Verification items for the finished model (mm, model axes). Face numbers are marked on the shaded views. Give positions to 0.01 mm unless a question says otherwise; leave off trailing zeros. Order: outer loops, then holes, each group sorted by start corner. A loop starts at its lowest first (then second) coordinate and runs counter-clockwise, first axis right, second up. Notation, with made-up numbers: (-24, 87) - (-12, 87) arc R9 ccw to (-12, 97) - close; hole circle Ø6 at (89.5, 89.5). An arc over 180 degrees is marked (long way). Answer as a JSON object with one key per item and string values.
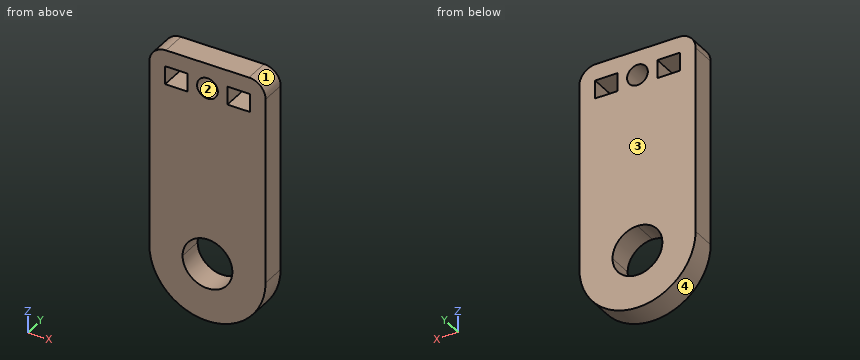
```python
from build123d import *

# Parameters (mm, degrees)
EXTRUDE_2_DEPTH = 3
SKETCH_1_4_W    = 2.7
SKETCH_1_4_H    = 2.2
SKETCH_1_4_R    = 1.25
EXTRUDE_3_DEPTH = 3
FILLET_2_R      = 2


with BuildPart() as part:
    # Sketch 1 → Extrude 2 (new body)
    with BuildSketch(Plane(origin=(0, 0, 0), x_dir=(1, 0, 0), z_dir=(0, 1, 0))):
        with BuildLine():
            ThreePointArc((-3, 12.25), (0, 15.25), (3, 12.25))
            Line((3, 12.25), (7, 12.25))
            ThreePointArc((7, 12.25), (0, 19.25), (-7, 12.25))
            Line((-7, 12.25), (-3, 12.25))
        make_face()
        with BuildLine():
            ThreePointArc((3, 12.25), (2.121320344, 10.128679656), (0, 9.25))
            Line((0, 9.25), (0, 5.25))
            ThreePointArc((0, 5.25), (4.949747468, 7.300252532), (7, 12.25))
            Line((7, 12.25), (3, 12.25))
        make_face()
        with BuildLine():
            Line((0, 5.25), (0, 9.25))
            ThreePointArc((0, 9.25), (-2.121320344, 10.128679656), (-3, 12.25))
            Line((-3, 12.25), (-7, 12.25))
            ThreePointArc((-7, 12.25), (-4.949747468, 7.300252532), (0, 5.25))
        make_face()
    extrude(amount=EXTRUDE_2_DEPTH)

    # Sketch 1_4 → Extrude 3 (add)
    with BuildSketch(Plane(origin=(0, 0, 0), x_dir=(1, 0, 0), z_dir=(0, 1, 0))):
        with BuildLine():
            ThreePointArc((7, 12.25), (4.949747468, 7.300252532), (0, 5.25))
            ThreePointArc((0, 5.25), (-4.949747468, 7.300252532), (-7, 12.25))
            Line((-7, 12.25), (-7, -12.25))
            Line((-7, -12.25), (7, -12.25))
            Line((7, -12.25), (7, 12.25))
        make_face()
        with Locations((-3.75, -9.170716156)):
            Rectangle(SKETCH_1_4_W, SKETCH_1_4_H, mode=Mode.SUBTRACT)
        with Locations((0, -9.25)):
            Circle(SKETCH_1_4_R, mode=Mode.SUBTRACT)
        with Locations((3.75, -9.170716156)):
            Rectangle(SKETCH_1_4_W, SKETCH_1_4_H, mode=Mode.SUBTRACT)
    extrude(amount=EXTRUDE_3_DEPTH)

    # Fillet 2
    fillet_2_edges = [part.edges().sort_by_distance(p)[0] for p in [
        (-7, 1.5, 12.25),
        (7, 1.5, 12.25),
    ]]
    fillet(fillet_2_edges, radius=FILLET_2_R)


solid = part.part
```
(1) Section check D-D (z = -10). Record the cut outline in (x, y), then the cut area to 3 significant figures.
Computed values:
{"outline": "(-7, 0) - (-1.98, 0) - (-1.98, 3) - (-7, 3) - close; (1.98, 0) - (7, 0) - (7, 3) - (1.98, 3) - close", "area": "30.1 mm²"}
(2) Release check for a two-part mould opening along X. For the marked faces 1, 2, 3 and 4 record: pulls with the +X half, pulls with the -X half, needs draft (parallel to the pull), parting line crosses it, or undercut.
Computed values:
{"face 1": "pulls with the +X half", "face 2": "undercut", "face 3": "needs draft", "face 4": "parting line crosses it"}
(3) Section check B-B (y = 2). Record the cut outline in (x, z), then the cut area to 3 significant figures.
Computed values:
{"outline": "(-7, -12.25) arc R7 ccw to (7, -12.25) - (7, 10.25) arc R2 ccw to (5, 12.25) - (-5, 12.25) arc R2 ccw to (-7, 10.25) - close; hole (-5.1, 8.07) - (-2.4, 8.07) - (-2.4, 10.27) - (-5.1, 10.27) - close; hole circle Ø6 at (0, -12.25); hole circle Ø2.5 at (0, 9.25); hole (2.4, 8.07) - (5.1, 8.07) - (5.1, 10.27) - (2.4, 10.27) - close", "area": "373 mm²"}
(4) Section check C-C (x = 0.5). Record the cut outline in (y, z), then the cut area to 3 significant figures.
Computed values:
{"outline": "(0, -19.23) - (3, -19.23) - (3, -15.21) - (0, -15.21) - close; (0, -9.29) - (3, -9.29) - (3, 8.1) - (0, 8.1) - close; (0, 10.4) - (3, 10.4) - (3, 12.25) - (0, 12.25) - close", "area": "69.8 mm²"}
(5) Material ranges on line 1 along Z through (x, y) = (0, 1.15); line 2 along X through (y, z) = (1.85, 9.25); line 3 along Z through (x, y) = (-1, 2.6), recorded low to high. Write a range as [from, to].
Computed values:
{"line 1": "z = [-19.25, -15.25], [-9.25, 8], [10.5, 12.25]", "line 2": "x = [-7, -5.1], [-2.4, -1.25], [1.25, 2.4], [5.1, 7]", "line 3": "z = [-19.18, -15.08], [-9.42, 8.5], [10, 12.25]"}
(6) Section check A-A (z = 9.25). Record the cut outline in (x, y), then the cut area to 3 significant figures.
Computed values:
{"outline": "(-7, 0) - (-5.1, 0) - (-5.1, 3) - (-7, 3) - close; (-2.4, 0) - (-1.25, 0) - (-1.25, 3) - (-2.4, 3) - close; (1.25, 0) - (2.4, 0) - (2.4, 3) - (1.25, 3) - close; (5.1, 0) - (7, 0) - (7, 3) - (5.1, 3) - close", "area": "18.3 mm²"}
(7) Gauge pin test, flat ends, axial feed: pin 1 Ø4 at (x, z) = (0, 9.25) entering from -Y; pin 2 Ø1 at (x, y) = (-5, 2) entering from -Z; pin 3 Ø1 at (x, y) = (-5.5, 1.5) entering from -Z; pin 4 Ø1 at (y, z) = (1, -14.5) entering from +X. Record the tip position at first contact, or that the pin passes through.
Computed values:
{"pin 1": "stops at y = 0", "pin 2": "stops at z = -17.61", "pin 3": "stops at z = -17.15", "pin 4": "stops at x = 6.78"}
